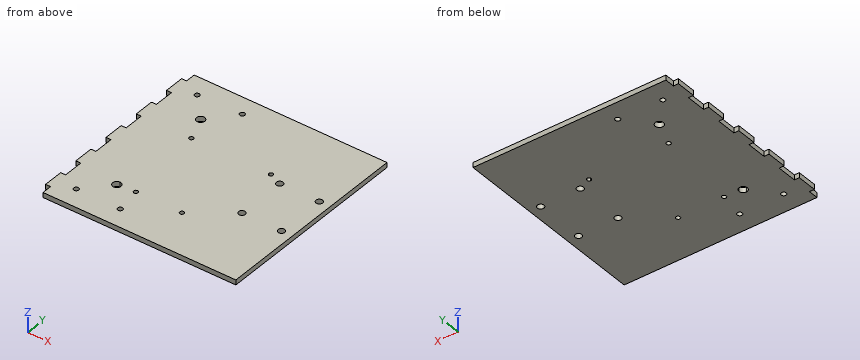
```python
from build123d import *

# Parameters (mm, degrees)
F0_R     = 1.5
F0_R_2   = 2
F0_R_3   = 2.5
F1_DEPTH = 3


with BuildPart() as f1:
    # F0 (on Top) → F1 (new body)
    with BuildSketch(Plane.XY):
        Polygon((74.5058632415, 0), (74.5058632415, 60), (-42.4941367585, 60), (-42.4941367585, 54), (-45.4941367585, 54), (-45.4941367585, 42), (-42.4941367585, 42), (-42.4941367585, 30), (-45.4941367585, 30), (-45.4941367585, 18), (-42.4941367585, 18), (-42.4941367585, 6), (-45.4941367585, 6), (-45.4941367585, -6), (-42.4941367585, -6), (-42.4941367585, -17.9991139914), (-45.4941367585, -17.9991139914), (-45.4941367585, -29.9991139914), (-42.4941367585, -29.9991139914), (-42.4941367585, -42), (-45.4941367585, -42), (-45.4941367585, -54), (-42.4941367585, -54), (-42.4941367585, -60), (74.5058632415, -60), align=None)
        with Locations((-31.4941367585, -48)):
            Circle(F0_R, mode=Mode.SUBTRACT)
        with BuildLine():
            ThreePointArc((-15.6229661617, -33.2851748408), (-16.3557725378, -35.053514937), (-18.1245875184, -35.785174315))
            ThreePointArc((-18.1245875184, -35.785174315), (-20.6229656359, -33.2835534841), (-18.1213448049, -30.7851753666))
            ThreePointArc((-18.1213448049, -30.7851753666), (-16.3546260654, -31.517981217), (-15.6229661617, -33.2851748408))
        make_face(mode=Mode.SUBTRACT)
        with BuildLine():
            ThreePointArc((-3.2708819532, -48), (-4.7708819532, -49.5), (-6.2708819532, -48))
            ThreePointArc((-6.2708819532, -48), (-4.7708819532, -46.5), (-3.2708819532, -48))
        make_face(mode=Mode.SUBTRACT)
        with BuildLine():
            Line((35.8920598827, 17.1), (35.8920598827, 0))
            Line((35.8920598827, 0), (35.8920598827, -32.4))
            Line((35.8920598827, -32.4), (21.9920598827, -32.4))
            ThreePointArc((21.9920598827, -32.4), (20.6920598827, -33.7), (19.3920598827, -32.4))
            Line((19.3920598827, -32.4), (-5.9079401173, -32.4))
            ThreePointArc((-5.9079401173, -32.4), (-7.2079401173, -33.7), (-8.5079401173, -32.4))
            Line((-8.5079401173, -32.4), (-12.4079401173, -32.4))
            Line((-12.4079401173, -32.4), (-12.4079401173, 17.1))
            ThreePointArc((-12.4079401173, 17.1), (-13.3271789328, 19.3192388155), (-11.1079401173, 18.4))
            Line((-11.1079401173, 18.4), (34.5920598827, 18.4))
            ThreePointArc((34.5920598827, 18.4), (35.8920598827, 19.7), (37.1920598827, 18.4))
            ThreePointArc((37.1920598827, 18.4), (36.8112986983, 17.4807611845), (35.8920598827, 17.1))
        make_face(mode=Mode.SUBTRACT)
        with Locations((43.8302124143, -15)):
            Circle(F0_R_2, mode=Mode.SUBTRACT)
        with Locations((67.8302124143, -15)):
            Circle(F0_R_2, mode=Mode.SUBTRACT)
        with Locations((-18.1229661617, 33.2851748408)):
            Circle(F0_R_3, mode=Mode.SUBTRACT)
        with Locations((-31.4937761504, 48)):
            Circle(F0_R, mode=Mode.SUBTRACT)
        with Locations((-4.7708819532, 48.8354042139)):
            Circle(F0_R, mode=Mode.SUBTRACT)
        with Locations((43.8302124143, 15)):
            Circle(F0_R_2, mode=Mode.SUBTRACT)
        with Locations((67.8302124143, 15)):
            Circle(F0_R_2, mode=Mode.SUBTRACT)
        with BuildLine():
            Line((35.8920598827, -32.4), (35.8920598827, 0))
            Line((35.8920598827, 0), (35.8920598827, 17.1))
            ThreePointArc((35.8920598827, 17.1), (34.9728210672, 17.4807611845), (34.5920598827, 18.4))
            Line((34.5920598827, 18.4), (-11.1079401173, 18.4))
            ThreePointArc((-11.1079401173, 18.4), (-11.4887013017, 17.4807611845), (-12.4079401173, 17.1))
            Line((-12.4079401173, 17.1), (-12.4079401173, -32.4))
            Line((-12.4079401173, -32.4), (-8.5079401173, -32.4))
            ThreePointArc((-8.5079401173, -32.4), (-7.2079401173, -31.1), (-5.9079401173, -32.4))
            Line((-5.9079401173, -32.4), (19.3920598827, -32.4))
            ThreePointArc((19.3920598827, -32.4), (20.6920598827, -31.1), (21.9920598827, -32.4))
            Line((21.9920598827, -32.4), (35.8920598827, -32.4))
        make_face()
    extrude(amount=F1_DEPTH)


solid = f1.part
```
Check sheet for the modelled part. Datum: model origin and axes. Units: mm. Give positions to 0.01 mm unless a question says otherwise; leave off trailing zeros. Loops run counter-clockwise (first coordinate to the right, second up) from the corner with the lowest first, then second, coordinate; pieces in that order, holes last. Notation, with made-up numbers: (49.5, 37) - (92.5, 37) arc R23 ccw to (92.5, 65) - close; hole circle Ø5 at (75.25, -20). An arc over 180 degrees is marked (long way). One line per question, with ' | ' between items. Start each with the question number.
1. Gauge pin test, flat ends, axial feed: pin 1 Ø0.9 at (x, z) = (-43.5, 2) entering from -Y; pin 2 Ø1.5 at (y, z) = (-12, 2) entering from -X. Record the tip position at first contact, or that the pin passes through.
2. Cross-section at B-B, the plane z = 1.2. Give the number of separate pieces and of enclosed holes in the cut face, plus the area to 3 significant figures.
3. Cross-section at A-A, the plane y = -15. Enter the section's corners in (x, z), plus the area to 3 significant figures.
4. Material ranges on line 1 along Y through (x, z) = (67.5, 2.65); line 2 along X through (y, z) = (18.4, 1.6); line 3 along Y through (x, z) = (-32, 0.6), recorded low to high. Write a range as [from, to].
Check result:
1) pin 1: stops at y = -54 | pin 2: stops at x = -42.49
2) separate pieces: 1 | enclosed holes: 14 | area: 14,100 mm2
3) outline: (-42.49, 0) - (41.83, 0) - (41.83, 3) - (-42.49, 3) - close; (45.83, 0) - (65.83, 0) - (65.83, 3) - (45.83, 3) - close; (69.83, 0) - (74.51, 0) - (74.51, 3) - (69.83, 3) - close | area: 327 mm2
4) line 1: y = [-60, -16.97], [-13.03, 13.03], [16.97, 60] | line 2: x = [-45.49, -13.71], [-11.11, 34.59], [37.19, 74.51] | line 3: y = [-60, -49.41], [-46.59, 46.59], [49.41, 60]
